from build123d import *

# Parameters (mm, degrees)
SKETCH_1_R          = 13
SKETCH_1_R_2        = 2
EXTRUDE_1_DEPTH     = 3
SKETCH_2_W          = 70
SKETCH_2_H          = 3
EXTRUDE_2_DEPTH     = 60
SKETCH_3_R          = 4.5
CUT_EXTRUDE_1_DEPTH = 87.040688049


with BuildPart() as part:
    # 草图1 → 凸台-拉伸1 (new body)
    with BuildSketch(Plane.XY):
        Polygon((-35, 22), (35, 22), (35, -28), (-35, -28), (-35, 0), align=None)
        Circle(SKETCH_1_R, mode=Mode.SUBTRACT)
        with Locations((0, 17.5)):
            Circle(SKETCH_1_R_2, mode=Mode.SUBTRACT)
        with Locations((17.5, 0)):
            Circle(SKETCH_1_R_2, mode=Mode.SUBTRACT)
        with Locations((0, -17.5)):
            Circle(SKETCH_1_R_2, mode=Mode.SUBTRACT)
        with Locations((-17.5, 0)):
            Circle(SKETCH_1_R_2, mode=Mode.SUBTRACT)
    extrude(amount=EXTRUDE_1_DEPTH)

    # 草图2 → 凸台-拉伸2 (add)
    with BuildSketch(Plane.XY.offset(3)):
        with Locations((0, -26.5)):
            Rectangle(SKETCH_2_W, SKETCH_2_H)
    extrude(amount=EXTRUDE_2_DEPTH)

    # 草图3 → 切除-拉伸1 (cut, through all)
    with BuildSketch(Plane(origin=(0, -25, 0), x_dir=(1, 0, 0), z_dir=(0, 1, 0))):
        with Locations(Location((21.213203436, -13.786796564, 0), (0, 0, 270))):
            Circle(SKETCH_3_R)
        with Locations(Location((21.213203436, -56.213203436, 0), (0, 0, 270))):
            Circle(SKETCH_3_R)
        with Locations(Location((-21.213203436, -56.213203436, 0), (0, 0, 270))):
            Circle(SKETCH_3_R)
        with Locations(Location((-21.213203436, -13.786796564, 0), (0, 0, 270))):
            Circle(SKETCH_3_R)
    extrude(amount=-CUT_EXTRUDE_1_DEPTH, mode=Mode.SUBTRACT)


solid = part.part
Here's how the part is built. I have some questions about the finished solid (model axes, mm). A direction names the side the tool comes from. Give positions to 0.01 mm unless a question says otherwise; leave off trailing zeros. Loops run counter-clockwise (first coordinate to the right, second up) from the corner with the lowest first, then second, coordinate; pieces in that order, holes last. Notation, with made-up numbers: (-23, -34.75) -> (-14, -34.75) arc R8 cw to (-14, -19.75) -> close; hole circle Ø6 at (-13, -31). An arc over 180 degrees is marked (long way). One line per item, written item: value.
Q1. Suppose I cut it at B-B on x = 0. Please give me the cut outline in (y, z).
Answers follow:
outline: (-28, 0) -> (-19.5, 0) -> (-19.5, 3) -> (-25, 3) -> (-25, 63) -> (-28, 63) -> close; (-15.5, 0) -> (-13, 0) -> (-13, 3) -> (-15.5, 3) -> close; (13, 0) -> (15.5, 0) -> (15.5, 3) -> (13, 3) -> close; (19.5, 0) -> (22, 0) -> (22, 3) -> (19.5, 3) -> close
Q2. We'd pull the mould along X, two halves only. Please class faces 3 (the face through (-35, -25.3, 22)), 4 (the face through (22.565, -26.479, 60.505)), 5 (the face through (-7, -12, 3)): pulls with the +X half, pulls with the -X half, needs draft (parallel to the pull), parting line crosses it, or undercut.
Answers follow:
face 3: pulls with the -X half
face 4: undercut
face 5: needs draft
Q3. Suppose I cut it at D-D on x = 11.5. Please give me the cut outline in (y, z).
Answers follow:
outline: (-28, 0) -> (-6.06, 0) -> (-6.06, 3) -> (-25, 3) -> (-25, 63) -> (-28, 63) -> close; (6.06, 0) -> (22, 0) -> (22, 3) -> (6.06, 3) -> close
Q4. I'm going to push flat-ended pins straight in: pin 1 Ø5 at (x, y) = (-7.5, -14) entering from +Z; pin 2 Ø8 at (x, y) = (5, -2) entering from +Z (3 decimals); pin 3 Ø18 at (x, z) = (6.5, 33) entering from +Y; pin 4 Ø5 at (x, y) = (-17.5, 0) entering from -Z. Where does each tip first touch, or does it pass through?
Answers follow:
pin 1: z = 3
pin 2: through
pin 3: y = -25
pin 4: z = 0
Q5. Suppose I cut it at A-A on y = 0. Please give me the cut outline in (x, z).
Answers follow:
outline: (-35, 0) -> (-19.5, 0) -> (-19.5, 3) -> (-35, 3) -> close; (-15.5, 0) -> (-13, 0) -> (-13, 3) -> (-15.5, 3) -> close; (13, 0) -> (15.5, 0) -> (15.5, 3) -> (13, 3) -> close; (19.5, 0) -> (35, 0) -> (35, 3) -> (19.5, 3) -> close
Q6. If I drill on line 1 along Y through (x, z) = (0, 2); line 2 along Z through (x, y) = (12, 18); line 3 along Y through (x, z) = (17, 1), over which ranges is the centre line in solid material (lowest first)?
Answers follow:
line 1: -28 to -19.5, -15.5 to -13, 13 to 15.5, 19.5 to 22
line 2: 0 to 3
line 3: -28 to -1.94, 1.94 to 22
Q7. On a 3-axis mill with a long thin cutter (end or side, diameter ignored), from which of +Z, -Z, +X, -X, +Y, -Y can I reach the whole of each face in a straight line? I mean faces 1 (the face through (0, -14, 0)), 2 (the face through (0, -25, 33)). Say none if no direction works.
Answers follow:
face 1: -Z, +X, -X, +Y, -Y
face 2: +Z, +X, -X, +Y
Q8. Suppose I cut it at C-C on y = 17.5. Please give me the cut outline in (x, z).
Answers follow:
outline: (-35, 0) -> (-2, 0) -> (-2, 3) -> (-35, 3) -> close; (2, 0) -> (35, 0) -> (35, 3) -> (2, 3) -> close
